Source: three-view drawing plus pictorial views. Frame: mm from the lowest corner of the part. Give positions to 0.01 mm unless a question says otherwise; leave off trailing zeros. Write each loop counter-clockwise with the first axis right and the second up, starting at its lowest first coordinate (ties: lowest second). Pieces come first, ordered by that corner, then holes.
Q1. Cut plane A-A on y = 62.5. Return the cut outline in (x, z).
Q2. Pin query (flat end, axial travel): pin 1 (3.5 mm diameter, centred on x = 33.25, y = 4, fed in from +Z); pin 2 (7 mm diameter, centred on x = 91.75, y = 4, fed in from -Z). Return the tip coordinate at first contact, or that it passes through.
Q3. Line query: L1, parallel to Y at x = 60, z = 3.3; L2, parallel to X at y = 87.5, z = 2.1; L3, parallel to Y at x = 35, z = 3.8. Output: solid intervals per line, ascending.
Q4. Cut plane B-B on x = 91.75. Return the cut outline in (y, z), plus the area to 4 significant figures.
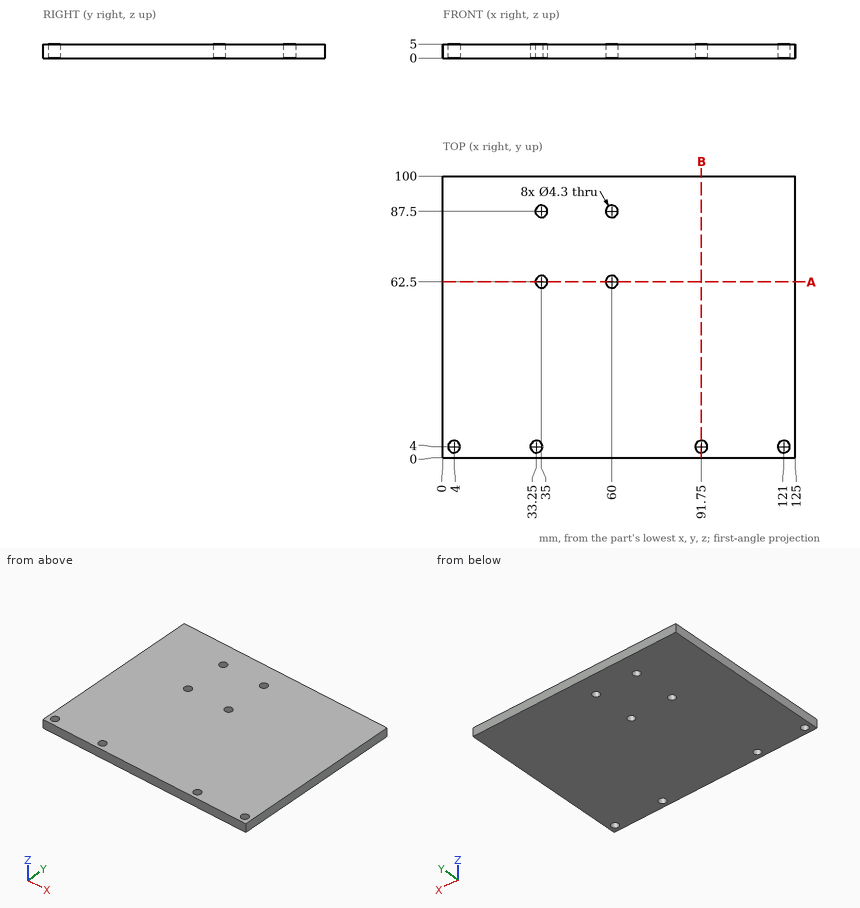
Data:
1. outline: (0, 0) - (32.85, 0) - (32.85, 5) - (0, 5) - close; (37.15, 0) - (57.85, 0) - (57.85, 5) - (37.15, 5) - close; (62.15, 0) - (125, 0) - (125, 5) - (62.15, 5) - close
2. pin 1: passes through
2. pin 2: stops at z = 0
3. L1: y = 0 to 60.35, 64.65 to 85.35, 89.65 to 100
3. L2: x = 0 to 32.85, 37.15 to 57.85, 62.15 to 125
3. L3: y = 0 to 2.75, 5.25 to 60.35, 64.65 to 85.35, 89.65 to 100
4. outline: (0, 0) - (1.85, 0) - (1.85, 5) - (0, 5) - close; (6.15, 0) - (100, 0) - (100, 5) - (6.15, 5) - close
4. area: 478.5 mm2
